from build123d import *

# Parameters (mm, degrees)
BOSS_EXTRUDE1_DEPTH = 1.5875
BOSS_EXTRUDE2_DEPTH = 25.4
BOSS_EXTRUDE3_START = -1.5875
BOSS_EXTRUDE3_DEPTH = 1.5875
SKETCH4_R           = 4.826
CUT_EXTRUDE1_DEPTH  = 55.9435


with BuildPart() as part:
    # Sketch1 → Boss-Extrude1 (new body)
    with BuildSketch(Plane(origin=(0, 0, 0), x_dir=(1, 0, 0), z_dir=(0, 1, 0))):
        with BuildLine():
            Line((-385.622421975, -25.4), (-9.24484395, -25.4))
            Line((-9.24484395, -25.4), (50.451144161, -75.490881607))
            ThreePointArc((50.451144161, -75.490881607), (68.343311232, -73.925519823), (66.777949447, -56.033352752))
            Line((66.777949447, -56.033352752), (0, 0))
            Line((0, 0), (-385.622421975, 0))
            Line((-385.622421975, 0), (-385.622421975, -25.4))
        make_face()
    extrude(amount=BOSS_EXTRUDE1_DEPTH)

    # Sketch2 → Boss-Extrude2 (add)
    with BuildSketch(Plane(origin=(0, 1.5875, 0), x_dir=(1, 0, 0), z_dir=(0, 1, 0))):
        with BuildLine():
            Line((-385.622421975, 0), (-385.622421975, -1.5875))
            Line((-385.622421975, -1.5875), (-1.332070664, -1.5875))
            Line((-1.332070664, -1.5875), (-1.02042533, -1.216095553))
            Line((-1.02042533, -1.216095553), (-0.577802747, -1.5875))
            Line((-0.577802747, -1.5875), (0, -1.5875))
            Line((0, -1.5875), (0, -2.072334072))
            Line((0, -2.072334072), (70.467441943, -61.201538616))
            ThreePointArc((70.467441943, -61.201538616), (68.950918532, -58.383132189), (66.777949447, -56.033352752))
            Line((66.777949447, -56.033352752), (0, 0))
            Line((0, 0), (-385.622421975, 0))
        make_face()
        with BuildLine():
            Line((-8.667041203, -23.8125), (-385.622421975, -23.8125))
            Line((-385.622421975, -23.8125), (-385.622421975, -25.4))
            Line((-385.622421975, -25.4), (-9.24484395, -25.4))
            Line((-9.24484395, -25.4), (50.451144161, -75.490881607))
            ThreePointArc((50.451144161, -75.490881607), (53.14255729, -77.222803492), (56.181487318, -78.226876364))
            Line((56.181487318, -78.226876364), (-8.667041203, -23.8125))
        make_face()
    extrude(amount=BOSS_EXTRUDE2_DEPTH)

    # Sketch3 → Boss-Extrude3 (add)
    with BuildSketch(Plane(origin=(0, 26.9875, 0), x_dir=(1, 0, 0), z_dir=(0, 1, 0)).offset(BOSS_EXTRUDE3_START)):
        with BuildLine():
            Line((-385.622421975, 0), (-385.622421975, -25.4))
            Line((-385.622421975, -25.4), (-9.24484395, -25.4))
            Line((-9.24484395, -25.4), (50.451144161, -75.490881607))
            ThreePointArc((50.451144161, -75.490881607), (68.343311232, -73.925519823), (66.777949447, -56.033352752))
            Line((66.777949447, -56.033352752), (0, 0))
            Line((0, 0), (-385.622421975, 0))
        make_face()
    extrude(amount=BOSS_EXTRUDE3_DEPTH)

    # Sketch4 → Cut-Extrude1 (cut)
    with BuildSketch(Plane(origin=(0, 26.9875, 0), x_dir=(1, 0, 0), z_dir=(0, 1, 0))):
        with Locations(Location((58.614546804, -65.76211718, 0), (0, 0, 270))):
            Circle(SKETCH4_R)
        with Locations(Location((-4.622421975, -12.7, 0), (0, 0, 270))):
            Circle(SKETCH4_R)
    extrude(amount=-CUT_EXTRUDE1_DEPTH, mode=Mode.SUBTRACT)


solid = part.part
Read the model definition and answer for the solid it produces. Units are mm, in the model's axes. A direction names the side the tool comes from. Give positions to 0.01 mm unless a question says otherwise; leave off trailing zeros. Write each loop counter-clockwise with the first axis right and the second up, starting at its lowest first coordinate (ties: lowest second). Pieces come first, ordered by that corner, then holes. Notation, with made-up numbers: M 46.25,8.25 L 57.25,8.25 A19 cw 57.25,41.25 Z; hole C 36.25,3.5 d2. An arc over 180 degrees is marked long. One line per item, written item: value. Start each with the question number.
(1) Find the intervals of material crossed by line 1 (Y direction, x = -51, z = 13); line 2 (Z direction, x = -204.5, y = 21); line 3 (X direction, y = 25.75, z = 16), in increasing order.
(2) Find section B-B (z = 12.7). Determine the outline of the cut face in (x, y).
(3) Find section C-C (z = 35). Determine the outline of the cut face in (x, y), plus the area to 3 significant figures.
(4) Find section A-A (x = -222.5). Determine the outline of the cut face in (y, z), plus the area to 3 significant figures.
(5) Flat-ended cylindrical pins translate along their axes: pin 1 Ø5 at (x, y) = (-320.5, 7.5) entering from +Z; pin 2 Ø5 at (y, z) = (24, 33.5) entering from +X; pin 3 Ø12 at (y, z) = (15, 42) entering from -X. Find the tip coordinate at first contact, or state that the pin passes through.
(6) A tool of negligible diameter and unlimited length cuts with its end or side. For faces 5 (the flat face through (34.74, 13.327, 31.223)), 6 (the flat face through (-200, 13, 25.4)), 7 (the flat face through (-195, 13, 23.812)), from which of +Z, -Z, +X, -X, +Y, -Y can it reach the whole face along a straight path? Write none if from no direction.
(7) Determine the mould class of faces 1 (the flat face through (-190, 13, 0)), 2 (the flat face through (20.185, 13.305, 50.095)), 3 (the flat face through (-158, 25.4, 17)), 4 (the flat face through (-158, 26.987, 22)) for opening direction Z: pulls with the +Z half, pulls with the -Z half, needs draft (parallel to the pull), parting line crosses it, or undercut.
(8) Find section D-D (z = 65.5). Determine the outline of the cut face in (x, y).
Results below:
1. line 1: y = 0 to 1.59, 25.4 to 26.99
1. line 2: z = 0 to 1.59, 23.81 to 25.4
1. line 3: x = -385.62 to -8.14, -1.1 to 19.07
2. outline: M -385.62,0 L -9.45,0 L -9.45,1.59 L -385.62,1.59 Z; M -385.62,25.4 L -9.45,25.4 L -9.45,26.99 L -385.62,26.99 Z; M 0.2,0 L 15.14,0 L 15.14,26.99 L 0.2,26.99 L 0.2,25.4 L 12.67,25.4 L 12.67,1.59 L 0.2,1.59 Z
3. outline: M 2.2,0 L 41.71,0 L 41.71,26.99 L 2.2,26.99 Z; hole M 4.67,1.59 L 39.24,1.59 L 39.24,25.4 L 4.67,25.4 Z
3. area: 243 mm^2
4. outline: M 0,0 L 26.99,0 L 26.99,25.4 L 0,25.4 Z; hole M 1.59,1.59 L 25.4,1.59 L 25.4,23.81 L 1.59,23.81 Z
4. area: 156 mm^2
5. pin 1: stops at z = 25.4
5. pin 2: stops at x = 42.9
5. pin 3: stops at x = 3.39
6. face 5: none
6. face 6: +Z, -X, +Y, -Y
6. face 7: -X
7. face 1: pulls with the -Z half
7. face 2: pulls with the +Z half
7. face 3: undercut
7. face 4: needs draft
8. outline: M 38.54,0 L 53.8,0 L 53.8,1.59 L 41.01,1.59 L 41.01,25.4 L 53.8,25.4 L 53.8,26.99 L 38.54,26.99 Z; M 63.43,0 L 71.31,0 L 71.31,1.59 L 63.43,1.59 Z; M 63.43,25.4 L 71.31,25.4 L 71.31,26.99 L 63.43,26.99 Z
